from build123d import *

# Parameters (mm, degrees)
F0_R      = 2.25
F1_DEPTH  = 0.8
F3_W      = 2.1
F3_H      = 16
F4_DEPTH  = 4.6
F5_DEPTH  = 5.5
F3_W_2    = 26.7
F3_H_2    = 1.8
F6_DEPTH  = 6.6
F3_H_3    = 14.6
F7_DEPTH  = 6.65
F9_W      = 3.6
F9_H      = 7.2
F10_DEPTH = 7
F12_W     = 3.3
F12_H     = 1.75
F12_H_2   = 1.65
F16_DEPTH = 2.5
F17_DEPTH = 1.7
F18_R     = 0.5
F19_SIZE  = 0.5
F20_DEPTH = 2.8


with BuildPart() as f1:
    # F0 (on Top) → F1 (new body, symmetric)
    with BuildSketch(Plane.XY):
        with BuildLine():
            Line((-17.5, -21.7), (17.5, -21.7))
            ThreePointArc((17.5, -21.7), (19.4091883092, -20.9091883092), (20.2, -19))
            Line((20.2, -19), (20.2, 19))
            ThreePointArc((20.2, 19), (19.4091883092, 20.9091883092), (17.5, 21.7))
            Line((17.5, 21.7), (-17.5, 21.7))
            ThreePointArc((-17.5, 21.7), (-19.4091883092, 20.9091883092), (-20.2, 19))
            Line((-20.2, 19), (-20.2, -19))
            ThreePointArc((-20.2, -19), (-19.4091883092, -20.9091883092), (-17.5, -21.7))
        make_face()
        with Locations((-17.5, -19)):
            Circle(F0_R, mode=Mode.SUBTRACT)
        with Locations((17.5, -19)):
            Circle(F0_R, mode=Mode.SUBTRACT)
        with Locations((-17.5, 19)):
            Circle(F0_R, mode=Mode.SUBTRACT)
        with Locations((17.5, 19)):
            Circle(F0_R, mode=Mode.SUBTRACT)
    extrude(amount=F1_DEPTH, both=True)

    # F3 (on offset) → F4 (join)
    with BuildSketch(Plane.XY.offset(0.8)):
        with Locations((-1.05, -13.3)):
            Rectangle(F3_W, F3_H)
        Polygon((0, -5.3), (0, -21.3), (5.9, -21.3), (13.9, -21.3), (13.9, -5.3), align=None)
        with BuildLine():
            ThreePointArc((6.9, -12.45), (6.7535533906, -12.8035533906), (6.4, -12.95))
            ThreePointArc((6.4, -12.95), (6.0464466094, -12.0964466094), (6.9, -12.45))
        make_face(mode=Mode.SUBTRACT)
    extrude(amount=F4_DEPTH)

    # F3 (on offset) → F5 (join)
    with BuildSketch(Plane.XY.offset(0.8)):
        Polygon((-8.8, -17.2), (-4.8, -17.2), (-4.8, -12.2), (-12.8, -12.2), (-12.8, -17.2), align=None)
    extrude(amount=F5_DEPTH)

    # F3 (on offset) → F6 (join)
    with BuildSketch(Plane.XY.offset(0.8)):
        with Locations((0, 19.7)):
            Rectangle(F3_W_2, F3_H_2)
        Polygon((-13.35, 4.2), (-13.35, -4.8), (0, -4.8), (13.35, -4.8), (13.35, 4.2), align=None)
    extrude(amount=F6_DEPTH)

    # F3 (on offset) → F7 (join)
    with BuildSketch(Plane.XY.offset(0.8)):
        with Locations((0, 11.5)):
            Rectangle(F3_W_2, F3_H_3)
    extrude(amount=F7_DEPTH)

    # F9 (on offset) → F10 (join)
    with BuildSketch(Plane(origin=(0, 0, -0.8), x_dir=(1, 0, 0), z_dir=(0, 0, -1))):
        with Locations((-19.7, -10.6)):
            Rectangle(F9_W, F9_H)
        with Locations((-19.7, -0.4)):
            Rectangle(F9_W, F9_H)
        with Locations((-19.7, 9.8)):
            Rectangle(F9_W, F9_H)
    extrude(amount=F10_DEPTH)

    # F12 (on offset) → F13 (revolve)
    with BuildSketch(Plane(origin=(0, 0, -4.8), x_dir=(1, 0, 0), z_dir=(0, 0, -1))):
        with Locations((-22.65, 9.025)):
            Rectangle(F12_W, F12_H)
    revolve(axis=Axis((-22.65, -9.9, -4.8), (-1, 0, 0)))

    # F12 (on offset) → F14 (revolve)
    with BuildSketch(Plane(origin=(0, 0, -4.8), x_dir=(1, 0, 0), z_dir=(0, 0, -1))):
        with Locations((-22.65, -1.025)):
            Rectangle(F12_W, F12_H_2)
    revolve(axis=Axis((-22.65, 0.2, -4.8), (-1, 0, 0)))

    # F12 (on offset) → F15 (revolve)
    with BuildSketch(Plane(origin=(0, 0, -4.8), x_dir=(1, 0, 0), z_dir=(0, 0, -1))):
        with Locations((-22.65, -11.175)):
            Rectangle(F12_W, F12_H)
    revolve(axis=Axis((-22.65, 10.3, -4.8), (-1, 0, 0)))

    # F9 (on offset) → F16 (join)
    with BuildSketch(Plane(origin=(0, 0, -0.8), x_dir=(1, 0, 0), z_dir=(0, 0, -1))):
        with BuildLine():
            Line((0, 14.9), (0, 12.375))
            ThreePointArc((0, 12.375), (2.8461047943, 13.5538952057), (4.025, 16.4))
            ThreePointArc((4.025, 16.4), (2.8461047943, 19.2461047943), (0, 20.425))
            Line((0, 20.425), (0, 17.9))
            Line((0, 17.9), (1.5, 17.9))
            Line((1.5, 17.9), (1.5, 14.9))
            Line((1.5, 14.9), (0, 14.9))
        make_face()
        with BuildLine():
            ThreePointArc((0, 20.425), (-4.025, 16.4), (0, 12.375))
            Line((0, 12.375), (0, 14.9))
            Line((0, 14.9), (-1.5, 14.9))
            Line((-1.5, 14.9), (-1.5, 17.9))
            Line((-1.5, 17.9), (0, 17.9))
            Line((0, 17.9), (0, 20.425))
        make_face()
    extrude(amount=F16_DEPTH)

    # F9 (on offset) → F17 (join)
    with BuildSketch(Plane(origin=(0, 0, -0.8), x_dir=(1, 0, 0), z_dir=(0, 0, -1))):
        with BuildLine():
            Line((0, 12.375), (0, 11.4))
            ThreePointArc((0, 11.4), (3.5355339059, 12.8644660941), (5, 16.4))
            ThreePointArc((5, 16.4), (3.5355339059, 19.9355339059), (0, 21.4))
            Line((0, 21.4), (0, 20.425))
            ThreePointArc((0, 20.425), (2.8461047943, 19.2461047943), (4.025, 16.4))
            ThreePointArc((4.025, 16.4), (2.8461047943, 13.5538952057), (0, 12.375))
        make_face()
        with BuildLine():
            ThreePointArc((0, 21.4), (-5, 16.4), (0, 11.4))
            Line((0, 11.4), (0, 12.375))
            ThreePointArc((0, 12.375), (-4.025, 16.4), (0, 20.425))
            Line((0, 20.425), (0, 21.4))
        make_face()
    extrude(amount=F17_DEPTH)

    # F18
    f18_edges = [f1.edges().sort_by_distance(p)[0] for p in [
        (-5, -16.4, -2.5),
        (-4.025, -16.4, -3.3),
    ]]
    fillet(f18_edges, radius=F18_R)

    # F19
    f19_edges = [f1.edges().sort_by_distance(p)[0] for p in [
        (5.9, -21.3, 5.4),
        (13.9, -13.3, 5.4),
        (5.9, -5.3, 5.4),
        (-2.1, -13.3, 5.4),
        (5.9, -12.45, 5.4),
    ]]
    chamfer(f19_edges, length=F19_SIZE)

    # F9 (on offset) → F20 (join)
    with BuildSketch(Plane(origin=(0, 0, -0.8), x_dir=(1, 0, 0), z_dir=(0, 0, -1))):
        Polygon((0, 16.4), (0, 14.9), (1.5, 14.9), (1.5, 17.9), (0, 17.9), align=None)
        Polygon((-1.5, 14.9), (0, 14.9), (0, 16.4), (0, 17.9), (-1.5, 17.9), align=None)
    extrude(amount=F20_DEPTH)


solid = f1.part
Part model, mm, in its own coordinate system. A direction names the side the tool comes from. Coordinates: 2 decimals unless noted, no trailing zeros. Loops run counter-clockwise (first coordinate to the right, second up) from the corner with the lowest first, then second, coordinate; pieces in that order, holes last. Notation, with made-up numbers: M 15.25,7.25 L 67.25,7.25 A15 ccw 67.25,35.25 Z; hole C 85.25,5 d7. An arc over 180 degrees is marked long. Use a Markdown table: item, result. Add a question column.
Q1. Pin check, flat tips, straight feed: P1, Ø3, axis at x = -10.5, z = 5, coming from the -Y side; P2, Ø8, axis at y = 8.5, z = 3.5, coming from the -X side; P3, Ø2.5, axis at y = -15.5, z = 4, coming from the -X side; P4, Ø8, axis at x = -17.5, z = 6, coming from the +Y side. Stop position of each tip, or through.
Q2. Probe L1, parallel to Y at x = 6.4, z = 3.2; L2, parallel to Y at x = 17.5, z = -0.25; L3, parallel to X at y = -12.45, z = 2. List the from-to ranges inside material, lowest first.
Q3. Mould opens along Y. For faces 1 (the flat face through (-20, -13.4, -4)), 2 (the flat face through (-21.5, 11, -3)), 3 (the flat face through (0, 20.6, 4)), 4 (the flat face through (-24.3, 10, -5)) say: +Y half, -Y half, draft (parallel to the pull), parting line (faces both ways), or undercut.
Q4. Cut at A-A (z = 3). Write the cut outline in (x, y).
Q5. Cut at B-B (x = 9). Write the cut outline in (y, z).
Q6. Which spindle directions (+Z, -Z, +X, -X, +Y, -Y) get a long thin tool onto all of the face, cutting with end or side? Do faces 5 (the cylindrical face through (-22.9, -0.2, -3.2)), 6 (the flat face through (6.4, -12.4, 0.8)), 7 (the flat face through (-2.1, -13, 3)), 8 (the flat face through (-13.35, 8, 4)). Say none if no direction does.
Q7. Cut at D-D (y = -2). Write the cut outline in (x, z), and give its area (3 significant figures).
Q8. Cut at C-C (z = -4.8). Write the cut outline in (x, y).
Worked out:
| question | item | result |
|---|---|---|
| 1 | P1 | stops at y = -17.2 |
| 1 | P2 | stops at x = -20.2 |
| 1 | P3 | stops at x = -12.8 |
| 1 | P4 | passes through |
| 2 | L1 | y = -21.3 to -12.95, -11.95 to -5.3, -4.8 to 20.6 |
| 2 | L2 | y = -21.7 to -21.25, -16.75 to 16.75, 21.25 to 21.7 |
| 2 | L3 | x = -12.8 to -4.8, -2.1 to 5.9, 6.9 to 13.9 |
| 3 | face 1 | -Y half |
| 3 | face 2 | undercut |
| 3 | face 3 | +Y half |
| 3 | face 4 | draft |
| 4 | outline | M -13.35,-4.8 L 13.35,-4.8 L 13.35,20.6 L -13.35,20.6 Z; M -12.8,-17.2 L -4.8,-17.2 L -4.8,-12.2 L -12.8,-12.2 Z; M -2.1,-21.3 L 13.9,-21.3 L 13.9,-5.3 L -2.1,-5.3 Z; hole C 6.4,-12.45 d1 |
| 5 | outline | M -21.7,-0.8 L 21.7,-0.8 L 21.7,0.8 L 20.6,0.8 L 20.6,7.4 L 18.8,7.4 L 18.8,7.45 L 4.2,7.45 L 4.2,7.4 L -4.8,7.4 L -4.8,0.8 L -5.3,0.8 L -5.3,4.9 L -5.8,5.4 L -20.8,5.4 L -21.3,4.9 L -21.3,0.8 L -21.7,0.8 Z |
| 6 | face 5 | -X |
| 6 | face 6 | +Z |
| 6 | face 7 | +Z, -Y |
| 6 | face 8 | +Z, -X, +Y, -Y |
| 7 | outline | M -21.5,-7.8 L -17.9,-7.8 L -17.9,-0.8 L 20.2,-0.8 L 20.2,0.8 L 13.35,0.8 L 13.35,7.4 L -13.35,7.4 L -13.35,0.8 L -20.2,0.8 L -20.2,-0.8 L -21.5,-0.8 Z |
| 7 | area | 266 mm2 |
| 8 | outline | M -24.3,-11.65 L -21.5,-11.65 L -21.5,-13.4 L -17.9,-13.4 L -17.9,-6.2 L -21.5,-6.2 L -21.5,-8.15 L -24.3,-8.15 Z; M -24.3,-1.45 L -21.5,-1.45 L -21.5,-3.2 L -17.9,-3.2 L -17.9,4 L -21.5,4 L -21.5,1.85 L -24.3,1.85 Z; M -24.3,8.55 L -21.5,8.55 L -21.5,7 L -17.9,7 L -17.9,14.2 L -21.5,14.2 L -21.5,12.05 L -24.3,12.05 Z |
